Model file for the job. Use its own axes, mm. A direction names the side the tool comes from. Coordinates: 2 decimals unless noted, no trailing zeros. Order: outer loops, then holes, each group sorted by start corner. A loop starts at its lowest first (then second) coordinate and runs counter-clockwise, first axis right, second up.
Autodesk Fusion 360 part; units mm, degrees
sketch "Boceto1" plane through (0, 0, -56) normal (0, 0, -1) x (1, 0, 0)
  line L0 (-169, 102) -> (-31, 102)
  line L1 (-31, 102) -> (-31, 108)
  line L2 (-31, 108) -> (-169, 108)
  line L3 (-169, 108) -> (-169, 102)
  line L4 (-169, 108) -> (-31, 108)
  line L5 (-31, 108) -> (-31, -66)
  line L6 (-31, -66) -> (-169, -66)
  line L7 (-169, -66) -> (-169, 108)
  line L8 (-169, 102) -> (-169, -60)
  line L9 (-169, -66) -> (-31, -66)
  line L10 (-31, -60) -> (-31, 102)
sketch "Boceto2" plane through (0, 0, -62) normal (0, 0, -1) x (1, 0, 0)
  line L0 (-169, -66) -> (-31, -66)
  line L1 (-31, -66) -> (-31, 108)
  line L2 (-31, 108) -> (-169, 108)
  line L3 (-169, 108) -> (-169, -66)
  line L4 (-163, 102) -> (-37, 102)
  line L5 (-37, 102) -> (-37, -60)
  line L6 (-37, -60) -> (-163, -60)
  line L7 (-163, -60) -> (-163, 102)
  line L8 (-163, -60) -> (-163, 102)
  line L9 (-37, 102) -> (-37, -60)
  line L10 (-175, 102) -> (-25, 102)
  line L11 (-25, -60) -> (-175, -60)
extrude "Extruir1" add sketch "Boceto1" along normal blind 6
extrude "Extruir2" add sketch "Boceto2" along normal blind 6 contours L4 L5 L6 L7 L8 L9 L10 L11
Q1. Cut at B-B, the plane x = -143. List the corners of the cut face in (y, z), plus the area to 3 significant figures.
Established:
outline: (-108, -62) - (-102, -62) - (-102, -68) - (60, -68) - (60, -62) - (66, -62) - (66, -56) - (-108, -56) - close
area: 2,020 mm2
Q2. Drop flat-ended pins along their axis: P1, Ø5, axis at y = -53, z = -65, coming from the -X side; P2, Ø6.5, axis at x = -89, z = -66, coming from the -Y side; P3, Ø3, axis at x = -93.5, z = -66.5, coming from the +Y side. Give the stop position or say it passes through.
Established:
P1: stops at x = -163
P2: stops at y = -102
P3: stops at y = 60
Q3. Probe line 1 (X direction, y = 30, z = -66.75); line 2 (Y direction, x = -44.5, z = -63.25). List the from-to ranges inside material, lowest first.
Established:
line 1: x = -163 to -37
line 2: y = -102 to 60
Q4. Cut at A-A, the plane y = 22. List the corners of the cut face in (x, z).
Established:
outline: (-169, -62) - (-163, -62) - (-163, -68) - (-37, -68) - (-37, -62) - (-31, -62) - (-31, -56) - (-169, -56) - close
Q5. Which spindle directions (+Z, -Z, +X, -X, +Y, -Y) get a long thin tool onto all of the face, cutting with end or side? Do faces 1 (the face through (-163, -20, -65)), 2 (the face through (-101, -102, -65)), 3 (the face through (-37, -22, -65)), 4 (the face through (-99, 60, -65)). Say none if no direction does.
Established:
face 1: -Z, -X, +Y, -Y
face 2: -Z, +X, -X, -Y
face 3: -Z, +X, +Y, -Y
face 4: -Z, +X, -X, +Y
Q6. Cut at C-C, the plane z = -65.5. List the corners of the cut face in (x, y), plus the area to 3 significant figures.
Established:
outline: (-163, -102) - (-37, -102) - (-37, 60) - (-163, 60) - close
area: 20,400 mm2
